Work out the finished part from the listing and answer in its coordinate system (mm). Give positions to 0.01 mm unless a question says otherwise; leave off trailing zeros. Loops run counter-clockwise (first coordinate to the right, second up) from the corner with the lowest first, then second, coordinate; pieces in that order, holes last. Notation, with made-up numbers: M 31.5,-38 L 71.5,-38 A32 cw 71.5,-9 Z; hole C -32,13 d5. An arc over 180 degrees is marked long. Answer in a Markdown table with one row per item. Add a question column.
from build123d import *

# Parameters (mm, degrees)
F0_R     = 33
F1_DEPTH = 2
F2_R     = 2.5
F3_DEPTH = 25
F4_R     = 1


with BuildPart() as f1:
    # F0 (on Top) → F1 (new body)
    with BuildSketch(Plane.XY):
        Circle(F0_R)
    extrude(amount=F1_DEPTH)

    # F2 (on face) → F3 (cut)
    with BuildSketch(Plane.XY.offset(2)):
        with Locations((-24.5, 0)):
            Circle(F2_R)
        with Locations((24.5, 0)):
            Circle(F2_R)
    extrude(amount=-F3_DEPTH, mode=Mode.SUBTRACT)

    # F4
    f4_edges = [f1.edges().sort_by_distance(p)[0] for p in [
        (-33, 0, 2),
    ]]
    fillet(f4_edges, radius=F4_R)


solid = f1.part
(1) The mould has two halves that part along X. Classify faces 1 (the face through (30.5, -12.6, 0.5)), 2 (the face through (22, 0, 1)), 3 (the face through (0, 0, 2)): pulls with the +X half, pulls with the -X half, needs draft (parallel to the pull), parting line crosses it, or undercut.
(2) Consider line 1 along Y through (x, z) = (24.5, 1.35); line 2 along Y through (x, z) = (24.5, 0.9); line 3 along Z through (x, y) = (-29.5, 13). Determine where each line is inside the solid, lowest interval first. Write a range as from..to.
(3) This flat-tipped pin is pushed along its axis until it touches: P1, Ø3, axis at x = -24.5, y = 0, coming from the -Z side. Where does it stop, or does it pass through?
(4) Section B-B, the plane z = 1.3 is taken. Determine the outline of the cut face in (x, y).
(5) Section A-A, the plane y = 0 is taken. Determine the outline of the cut face in (x, z).
Numbers:
| question | item | result |
|---|---|---|
| 1 | face 1 | parting line crosses it |
| 1 | face 2 | undercut |
| 1 | face 3 | needs draft |
| 2 | line 1 | y = -22.01..-2.5, 2.5..22.01 |
| 2 | line 2 | y = -22.11..-2.5, 2.5..22.11 |
| 2 | line 3 | z = 0..1.97 |
| 3 | P1 | passes through |
| 4 | outline | C 0,0 d65.91; hole C -24.5,0 d5; hole C 24.5,0 d5 |
| 5 | outline | M -33,0 L -27,0 L -27,2 L -32,2 A1 ccw -33,1 Z; M -22,0 L 22,0 L 22,2 L -22,2 Z; M 27,0 L 33,0 L 33,1 A1 ccw 32,2 L 27,2 Z |
